Geometry: final body of the model. Coordinates: model frame, mm. Face numbers are marked on the shaded views. A direction names the side the tool comes from. Coordinates: 2 decimals unless noted, no trailing zeros. Order: outer loops, then holes, each group sorted by start corner. A loop starts at its lowest first (then second) coordinate and runs counter-clockwise, first axis right, second up. Notation, with made-up numbers: M 50,26.5 L 70,26.5 A17 ccw 70,48.5 Z; hole C 25.25,-21 d10. An arc over 180 degrees is marked long. Use CSV: the item, a comma, the result in double quotes. Start each with the question number.
1. Section query C-C on z = 6.5. Return the cut outline in (x, y), and give its area (3 significant figures).
2. Material intervals for line 1 (Y direction, x = 0, z = 1.2); line 2 (Z direction, x = -2.25, y = -1.5); line 3 (Y direction, x = -0.5, z = 1.75), sorted ascending.
3. Section query D-D on y = 1.5. Return the cut outline in (x, z), and give its area (3 significant figures).
4. Section query A-A on x = 0. Return the cut outline in (y, z).
5. Set-up query: the marked faces 1 and 2. Return all of +Z, -Z, +X, -X, +Y, -Y with unobstructed straight access to the full face (end or side cutting, diameter ignored); none if empty.
6. First-contact query: P1, Ø1.5, axis at x = 1, z = 21.5, coming from the +Y side. Flat tip, straight axial feed; report the tip coordinate or a pass-through.
from build123d import *

# Parameters (mm, degrees)
SKETCH1_R           = 2.2
BOSS_EXTRUDE1_DEPTH = 26
SKETCH2_R           = 3.5
BOSS_EXTRUDE2_DEPTH = 3
SKETCH3_R           = 1
CUT_EXTRUDE1_DEPTH  = 5


with BuildPart() as part:
    # Sketch1 → Boss-Extrude1 (new body)
    with BuildSketch(Plane.XY):
        with Locations(Location((0, 0, 0), (0, 0, 180))):
            Circle(SKETCH1_R)
    extrude(amount=BOSS_EXTRUDE1_DEPTH)

    # Sketch2 → Boss-Extrude2 (add)
    with BuildSketch(Plane.XY.offset(26)):
        Circle(SKETCH2_R)
    extrude(amount=-BOSS_EXTRUDE2_DEPTH)

    # Sketch3 → Cut-Extrude1 (cut)
    with BuildSketch(Plane(origin=(0, 0, 0), x_dir=(-1, 0, 0), z_dir=(0, 0, -1))):
        Circle(SKETCH3_R)
    extrude(amount=-CUT_EXTRUDE1_DEPTH, mode=Mode.SUBTRACT)


solid = part.part
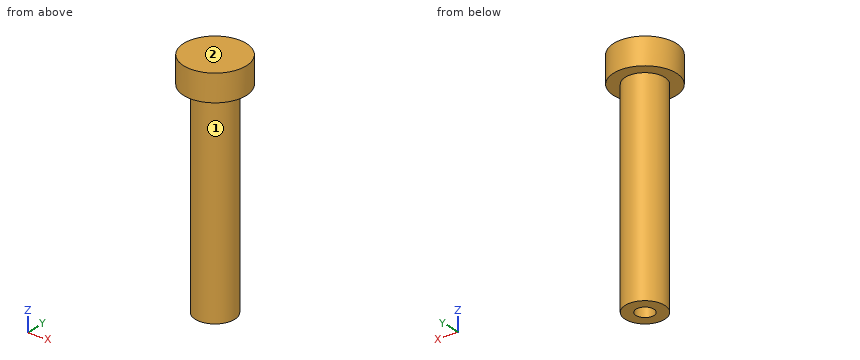
Results list:
1,outline,"C 0,0 d4.4"
1,area,"15.2 mm²"
2,line 1,"y = -2.2 to -1, 1 to 2.2"
2,line 2,"z = 23 to 26"
2,line 3,"y = -2.14 to -0.87, 0.87 to 2.14"
3,outline,"M -3.16,23 L -1.61,23 L -1.61,0 L 1.61,0 L 1.61,23 L 3.16,23 L 3.16,26 L -3.16,26 Z"
3,area,"93.0 mm²"
4,outline,"M -3.5,23 L -2.2,23 L -2.2,0 L -1,0 L -1,5 L 1,5 L 1,0 L 2.2,0 L 2.2,23 L 3.5,23 L 3.5,26 L -3.5,26 Z"
5,face 1,"-Z"
5,face 2,"+Z, +X, -X, +Y, -Y"
6,P1,"stops at y = 2.19"
